Verification items for the finished model (mm, model axes). A direction names the side the tool comes from. Round coordinates to 2 decimals unless told otherwise and drop trailing zeros. Write each loop counter-clockwise with the first axis right and the second up, starting at its lowest first coordinate (ties: lowest second). Pieces come first, ordered by that corner, then holes. Notation, with made-up numbers: (65.5, -5.75) - (73.5, -5.75) arc R13 cw to (73.5, 3.25) - close; hole circle Ø4 at (82.25, -8.75). An arc over 180 degrees is marked (long way). Answer as a JSON object with one key per item and string values. Group by question number.
1) Go/stop test with flat-tipped pins: pin 1 Ø6.5 at (x, y) = (-1.5, 2.5) entering from -Z; pin 2 Ø3 at (y, z) = (2.5, 7) entering from +X; pin 3 Ø10.5 at (x, z) = (20, -47.5) entering from +Y. Record where each tip stops, or that it passes through.
2) Section check B-B (y = 8). State how many separate pieces and enclosed holes the cut face has, then the cut area to 3 significant figures.
3) Section check A-A (z = 30). Enter the section's corners in (x, y), then the cut area to 3 significant figures.
4) Section check D-D (z = -8). Enter the section's corners in (x, y).
5) Mould release check, pull along X, two halves, no side actions. Record for faces 1 (the flat face through (0, 8, -72.5)), 2 (the cylindrical face through (0.138, 8.465, 65.647)), 3 (the cylindrical face through (15, 5, 24)), 4 (the flat face through (-35, 8, -1)): +X half, -X half, draft (parallel to the pull), parting line (faces both ways), or undercut.
6) Set-up check for faces 5 (the cylindrical face through (-15, 5, 36)), 6 (the flat face through (0, 3, -55)), 7 (the flat face through (0, 0, -1)), 8 (the flat face through (30, 3, 1)), 9 (the cylindrical face through (-22.55, 6.91, 53.64)): record each of +Z, -Z, +X, -X, +Y, -Y from which the full face is reachable in a straight line by a thin tool's end or side.
7) Thickness scan on line 1 (X direction, y = 4.5, z = 29.5); line 2 (X direction, y = 6.25, z = 47.5); line 3 (Z direction, x = 15.5, y = 1.75). Record the ranges inside material, lowest first.
8) Section check C-C (z = 62.5). Enter the section's corners in (x, y), then the cut area to 4 significant figures.
```python
from build123d import *

# Parameters (mm, degrees)
SKETCH_1_R          = 4.1
SKETCH_1_R_2        = 6
EXTRUDE_1_DEPTH     = 11
SKETCH_2_R          = 6.65
CUT_EXTRUDE_1_DEPTH = 8.3
EXTRUDE_START       = -6
SKETCH_3_W          = 70
SKETCH_3_H          = 145
SKETCH_3_R          = 3.15
EXTRUDE_2_DEPTH     = 5


with BuildPart() as part:
    # 草图1 → 凸台-拉伸1 (new body)
    with BuildSketch(Plane(origin=(0, 0, 0), x_dir=(1, 0, 0), z_dir=(0, 1, 0))):
        with BuildLine():
            Line((-28, -55), (28, -55))
            ThreePointArc((28, -55), (29.414213562, -54.414213562), (30, -53))
            Line((30, -53), (30, 53))
            ThreePointArc((30, 53), (29.414213562, 54.414213562), (28, 55))
            Line((28, 55), (-28, 55))
            ThreePointArc((-28, 55), (-29.414213562, 54.414213562), (-30, 53))
            Line((-30, 53), (-30, -53))
            ThreePointArc((-30, -53), (-29.414213562, -54.414213562), (-28, -55))
        make_face()
        with Locations(Location((-20, 47.5, 0), (0, 0, 270))):
            Circle(SKETCH_1_R, mode=Mode.SUBTRACT)
        with Locations(Location((20, 47.5, 0), (0, 0, 90))):
            Circle(SKETCH_1_R, mode=Mode.SUBTRACT)
        with Locations(Location((-20, -47.5, 0), (0, 0, 90))):
            Circle(SKETCH_1_R, mode=Mode.SUBTRACT)
        with Locations(Location((20, -47.5, 0), (0, 0, 270))):
            Circle(SKETCH_1_R, mode=Mode.SUBTRACT)
        with Locations(Location((-15, 30, 0), (0, 0, 270))):
            Circle(SKETCH_1_R_2, mode=Mode.SUBTRACT)
        with Locations(Location((15, 30, 0), (0, 0, 90))):
            Circle(SKETCH_1_R_2, mode=Mode.SUBTRACT)
        with Locations(Location((15, -30, 0), (0, 0, 270))):
            Circle(SKETCH_1_R_2, mode=Mode.SUBTRACT)
        with Locations(Location((-15, -30, 0), (0, 0, 90))):
            Circle(SKETCH_1_R_2, mode=Mode.SUBTRACT)
    extrude(amount=EXTRUDE_1_DEPTH)

    # 草图2 → 切除-拉伸1 (cut)
    with BuildSketch(Plane(origin=(0, 11, 0), x_dir=(1, 0, 0), z_dir=(0, 1, 0))):
        with Locations(Location((-20, 47.5, 0), (0, 0, 270))):
            Circle(SKETCH_2_R)
        with Locations(Location((-20, -47.5, 0), (0, 0, 270))):
            Circle(SKETCH_2_R)
        with Locations(Location((20, 47.5, 0), (0, 0, 270))):
            Circle(SKETCH_2_R)
        with Locations(Location((20, -47.5, 0), (0, 0, 270))):
            Circle(SKETCH_2_R)
    extrude(amount=-CUT_EXTRUDE_1_DEPTH, mode=Mode.SUBTRACT)

    # 草图3 → 凸台-拉伸2 (add)
    with BuildSketch(Plane.XZ.offset(EXTRUDE_START)):
        Rectangle(SKETCH_3_W, SKETCH_3_H)
        with Locations(Location((-25, 62.5, 0), (0, 0, 270))):
            Circle(SKETCH_3_R, mode=Mode.SUBTRACT)
        with Locations(Location((25, 62.5, 0), (0, 0, 270))):
            Circle(SKETCH_3_R, mode=Mode.SUBTRACT)
        with Locations(Location((25, -62.5, 0), (0, 0, 270))):
            Circle(SKETCH_3_R, mode=Mode.SUBTRACT)
        with Locations(Location((-25, -62.5, 0), (0, 0, 270))):
            Circle(SKETCH_3_R, mode=Mode.SUBTRACT)
        with Locations(Location((0, 62.5, 0), (0, 0, 270))):
            Circle(SKETCH_3_R, mode=Mode.SUBTRACT)
        with Locations(Location((0, -62.5, 0), (0, 0, 270))):
            Circle(SKETCH_3_R, mode=Mode.SUBTRACT)
        with BuildLine():
            Line((-30, 53), (-30, -53))
            ThreePointArc((-30, -53), (-29.414213562, -54.414213562), (-28, -55))
            Line((-28, -55), (28, -55))
            ThreePointArc((28, -55), (29.414213562, -54.414213562), (30, -53))
            Line((30, -53), (30, 53))
            ThreePointArc((30, 53), (29.414213562, 54.414213562), (28, 55))
            Line((28, 55), (-28, 55))
            ThreePointArc((-28, 55), (-29.414213562, 54.414213562), (-30, 53))
        make_face(mode=Mode.SUBTRACT)
    extrude(amount=-EXTRUDE_2_DEPTH)


solid = part.part
```
Returned:
{
 "1": {"pin 1": "z = -55", "pin 2": "x = 30", "pin 3": "y = 2.7"},
 "2": {"separate pieces": "1", "enclosed holes": "14", "area": "8,950 mm2"},
 "3": {"outline": "(-35, 6) - (-30, 6) - (-30, 0) - (-21, 0) - (-21, 11) - (-35, 11) - close; (-9, 0) - (9, 0) - (9, 11) - (-9, 11) - close; (21, 0) - (30, 0) - (30, 6) - (35, 6) - (35, 11) - (21, 11) - close", "area": "446 mm2"},
 "4": {"outline": "(-35, 6) - (-30, 6) - (-30, 0) - (30, 0) - (30, 6) - (35, 6) - (35, 11) - (-35, 11) - close"},
 "5": {"face 1": "draft", "face 2": "undercut", "face 3": "undercut", "face 4": "-X half"},
 "6": {"face 5": "+Y, -Y", "face 6": "-Z, +X, -X, -Y", "face 7": "+Z, -Z, +X, -X, -Y", "face 8": "+Z, -Z, +X, -Y", "face 9": "+Y"},
 "7": {"line 1": "-30 to -20.98, -9.02 to 9.02, 20.98 to 30", "line 2": "-35 to -26.65, -13.35 to 13.35, 26.65 to 35", "line 3": "-55 to -35.98, -24.02 to 24.02, 35.98 to 55"},
 "8": {"outline": "(-35, 6) - (-28.15, 6) - (-28.15, 11) - (-35, 11) - close; (-21.85, 6) - (-3.15, 6) - (-3.15, 11) - (-21.85, 11) - close; (3.15, 6) - (21.85, 6) - (21.85, 11) - (3.15, 11) - close; (28.15, 6) - (35, 6) - (35, 11) - (28.15, 11) - close", "area": "255.5 mm2"}
}
